The listing builds one solid part. Answer for the finished solid, in the listing's coordinates (mm). Give positions to 0.01 mm unless a question says otherwise; leave off trailing zeros. Order: outer loops, then holes, each group sorted by start corner. A loop starts at its lowest first (then second) coordinate and runs counter-clockwise, first axis right, second up. Notation, with made-up numbers: (-9, 8.5) - (36, 8.5) arc R28 cw to (36, 42.5) - close; hole circle Ø1 at (35, 55.25). An arc over 180 degrees is marked (long way). Use a Markdown table: item, result. Add a question column.
1) Find section A-A, the plane x = 3.5. Determine the outline of the cut face in (y, z), plus the area to 3 significant figures.
2) Flat-ended cylindrical pins translate along their axes: pin 1 (5 mm diameter, centred on y = 0, z = 0, fed in from +X); pin 2 (2 mm diameter, centred on x = 6.5, z = 6, fed in from -Y). Find the tip coordinate at first contact, or state that the pin passes through.
3) The mould has two halves that part along Y. Classify faces 1 (the face through (4.591, -2.83, 3.087)), 2 (the face through (9.3, -0.1, -5.2)), 3 (the face through (4.585, -6.961, 3.944)), 4 (the face through (4.585, 6.961, -3.944)): released by +Y, released by -Y, zero draft, split by the parting line, or undercut.
4) Straight lines are drawn through the part: line 1 (Z direction, x = 3.25, y = 0); line 2 (Z direction, x = 7, y = 3); line 3 (Y direction, x = 1.5, z = -1). For each, find the intervals that lie inside material, in ascending order.
Autodesk Inventor part; units mm, degrees
ref_plane "Work Plane1" through (-16.85, 0, 0) normal (0, -0.866, -0.5) x (1, 0, 0)
ref_plane "YZ Plane" through (0, 0, 0) normal (1, 0, 0) x (0, 1, 0)
ref_plane "XZ Plane" through (0, 0, 0) normal (0, 1, 0) x (-1, 0, 0)
sketch "草图1" plane through (0, 0, 0) normal (1, 0, 0) x (0, 1, 0)
  line L0 (-9.2376, 0) -> (-4.6188, 8)
  line L1 (-4.6188, 8) -> (4.6188, 8)
  line L2 (4.6188, 8) -> (9.2376, 0)
  line L3 (9.2376, 0) -> (4.6188, -8)
  line L4 (4.6188, -8) -> (-4.6188, -8)
  line L5 (-4.6188, -8) -> (-9.2376, 0)
  point P0 (0, 0)
  point P1 (0, 0)
  dimension "d0" = 18.4752
extrude "轴承体" add sketch "草图1" along normal blind 9.3
sketch "草图2" plane through (0, 0, 0) normal (0, 0, 1) x (1, 0, 0)
  line L0 (0, 4.6188) -> (0, 9.2376)
  line L1 (0, 9.2376) -> (9.3, 9.2376)
  line L2 (9.3, 4.6188) -> (9.3, 9.2376)
  line L3 (-1.86, 0) -> (11.16, 0)
  line L4 (0.7145, 9.2376) -> (0, 8)
  line L5 (8.5855, 9.2376) -> (9.3, 8)
  dimension "d3" = 30
  dimension "d4" = 30
  dimension "d5" = 16
  dimension "d6" = 16
revolve "倒角1" cut sketch "草图2" angle 360 about axis through (-10, 0, 0) along (1, 0, 0)
sketch "草图3" plane through (9.3, 0, 0) normal (1, 0, 0) x (0, 0, -1)
  arc A0 (-4, -6.9282) -> (4, -6.9282) centre (0, 0) ccw
hole "螺纹" at (9.3, 0, 0) direction (-1, 0, 0) diameter 8.376 end through all
chamfer "倒角2" distance 0.8119 angle 30 1 edges at (9.3, 0, 4.188) measured on face at (9.3, 6.6899, -0.1683)
chamfer "倒角3" distance 0.8119 angle 30 1 edges at (0, 0, 4.188) measured on face at (0, 6.6899, -0.1683)
ref_plane "Work Plane1" through (-16.85, 0, 0) normal (0, -0.866, -0.5) x (1, 0, 0)
equation "\"d0\" = 1.1547 * SW"
equation "\"d1\" = KOH"
equation "\"d3\" = ANG1"
equation "\"d4\" = ANG2"
equation "\"d5\" = SW0"
equation "\"d6\" = SW01"
equation "\"d8\" = -0.5 * GD1 + 0.5 * NND"
equation "\"d40\" = -0.5 * GD1 + 0.5 * NND"
equation "\"d10\" = -0.5 * GD1 + 0.5 * NND"
equation "\"d41\" = -0.5 * GD1 + 0.5 * NND"
equation "\"ANG1\" = 30deg"
equation "\"ANG2\" = 30deg"
equation "\"KOH\" = 9.3"
equation "\"SW\" = 16"
equation "\"SW0\" = SW"
equation "\"SW01\" = SW"
equation "\"GUL\" = 0.541266 * PTC"
equation "\"TOA\" = 30deg"
equation "\"PTC\" = 1.5"
equation "\"E0\" = 1.155 * SW"
equation "\"GAL\" = 0.541266 * PTC"
properties part number "螺母 GB/T 6175 M10" material "钢，软"
The answers:
| question | item | result |
|---|---|---|
| 1 | outline | (-9.24, 0) - (-4.62, -8) - (4.62, -8) - (9.24, 0) - (4.62, 8) - (-4.62, 8) - close; hole circle Ø8.38 at (0, 0) |
| 1 | area | 167 mm2 |
| 2 | pin 1 | through |
| 2 | pin 2 | y = -6.35 |
| 3 | face 1 | undercut |
| 3 | face 2 | zero draft |
| 3 | face 3 | released by -Y |
| 3 | face 4 | released by +Y |
| 4 | line 1 | -8 to -4.19, 4.19 to 8 |
| 4 | line 2 | -8 to -2.92, 2.92 to 8 |
| 4 | line 3 | -8.66 to -4.07, 4.07 to 8.66 |
